The figure shows three views and two pictorial views of one solid part (mm, origin at its lowest corner). Answer the questions. A direction names the side the tool comes from. Coordinates: 2 decimals unless noted, no trailing zeros. Order: outer loops, then holes, each group sorted by start corner. A loop starts at its lowest first (then second) coordinate and runs counter-clockwise, first axis right, second up. Notation, with made-up numbers: (-27.75, -9.75) - (31.25, -9.75) arc R10 ccw to (31.25, 9.25) - close; hole circle Ø3 at (24.25, 34.5). An arc over 180 degrees is marked (long way). Use one line per item in the form item = value. Start each with the question number.
Item 1: A tool of negligible diameter and unlimited length cuts with its end or side. For the marked faces 1 and 2, from which of +Z, -Z, +X, -X, +Y, -Y can it reach the whole face along a straight path? Write none if from no direction.
Item 2: Consider line 1 along X through (y, z) = (1.95, 12.7); line 2 along Y through (x, z) = (55.05, 12.7); line 3 along Z through (x, y) = (25.4, 2.3). Determine where each line is inside the solid, lowest interval first. Write a range as [from, to].
Item 3: Section C-C, the plane z = 12.7 is taken. Count the separate pieces of the cut face and the enclosed holes in it.
Item 4: Each of these flat-tipped pins is pushed along its axis until it touches: pin 1 Ø3 at (y, z) = (18.5, 3.5) entering from -X (3 decimals); pin 2 Ø6 at (x, z) = (25.4, 12.7) entering from +Y (3 decimals). Where does it stop, or does it pass through?
Item 5: Section B-B, the plane x = 25.4 is taken. Write down the section's boundary in (y, z) (1 decimal).
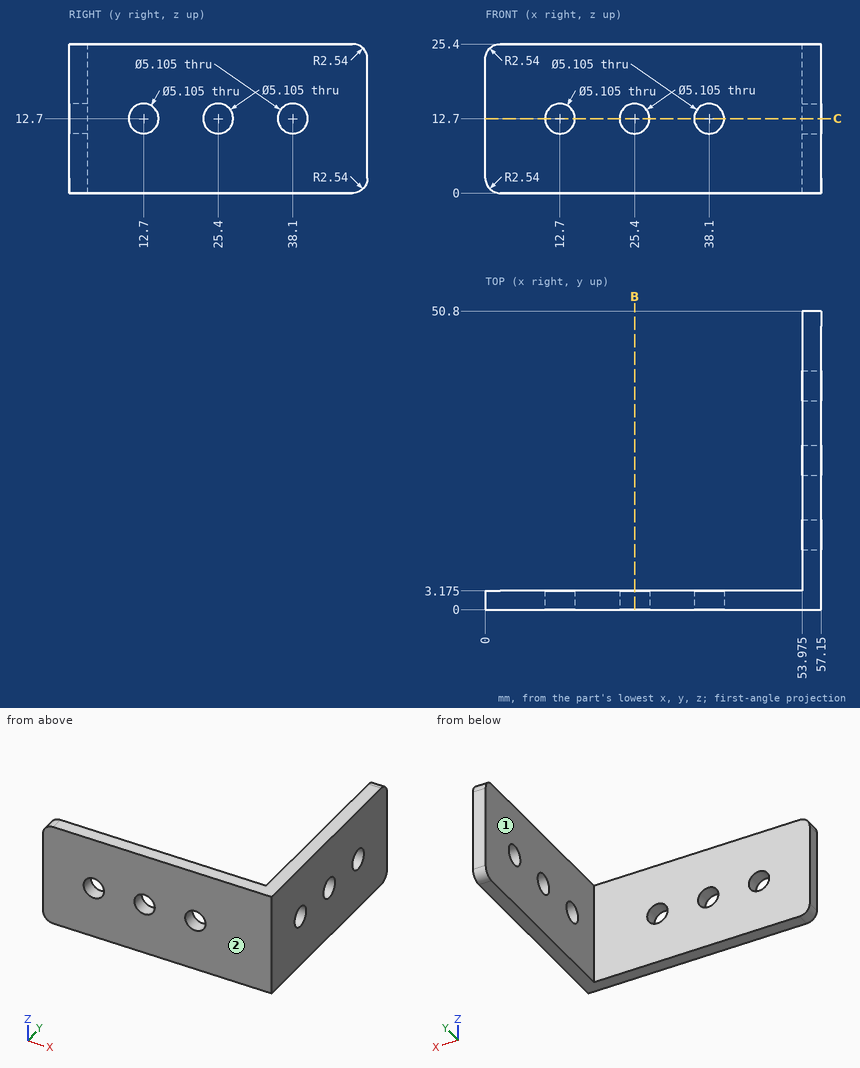
Response:
q1.face_1 = +Z, -Z, -X, +Y
q1.face_2 = +Z, -Z, +X, -X, -Y
q2.line_1 = [0, 10.15], [15.25, 22.85], [27.95, 35.55], [40.65, 57.15]
q2.line_2 = [0, 10.15], [15.25, 22.85], [27.95, 35.55], [40.65, 50.8]
q2.line_3 = [0, 10.15], [15.25, 25.4]
q3.separate_pieces = 7
q3.enclosed_holes = 0
q4.pin_1 = 53.975
q4.pin_2 = 3.175
q5.outline = (0, 0) - (3.2, 0) - (3.2, 10.1) - (0, 10.1) - close; (0, 15.3) - (3.2, 15.3) - (3.2, 25.4) - (0, 25.4) - close
